Input: part model. Units: mm. Frame: model coordinates. A direction names the side the tool comes from. Coordinates: 2 decimals unless noted, no trailing zeros. Write each loop counter-clockwise with the first axis right and the second up, starting at its lowest first coordinate (ties: lowest second). Pieces come first, ordered by that corner, then holes. Notation, with made-up numbers: (76.25, -36) - (107.25, -36) arc R25 cw to (107.25, -12) - close; hole circle Ø9 at (58, -39). An arc over 180 degrees is marked (long way). Use a Markdown table: item, result. Add a question column.
Q1. Pin query (flat end, axial travel): P1, Ø1, axis at x = -8, y = 6, coming from the -Z side; P2, Ø8, axis at x = -5, z = -1, coming from the -Y side; P3, Ø1.5, axis at x = -14, z = -21, coming from the +Y side; P4, Ø0.9, axis at x = 3.5, y = 3.5, coming from the +Z side. Return the tip coordinate at first contact, or that it passes through.
Q2. Section query D-D (y = 5.5). Return the cut outline in (x, z), then the cut area to 3 significant figures.
Q3. Section query A-A (z = -25.5). Return the cut outline in (x, y), then the cut area to 3 significant figures.
Q4. Material intervals for probe 1 along X at (y, z) = (14.5, -9); probe 2 along X at (y, z) = (7, -21.5); probe 3 along Z at (x, y) = (-4.25, 9.5), sorted ascending. Write a range as from..to.
Q5. Mould query, pull axis X, two halves, no side actions, for faces 1 (the face through (-13, 8.85, -22)), 2 (the face through (5.347, 4, -22)), 3 (the face through (-5, 7, 0)). Classes: released by +X, released by -X, zero draft, split by the parting line, or undercut.
Q6. Set-up query: faces 4 (the face through (-5, 7, -12.127)), 5 (the face through (-14, 4, -14.627)), 6 (the face through (2.5, 7, -6)), 7 (the face through (-10.624, 4, -22)). Return all of +Z, -Z, +X, -X, +Y, -Y with unobstructed straight access to the full face (end or side cutting, diameter ignored); none if empty.
Q7. Section query B-B (y = 12.5). Return the cut outline in (x, z), then the cut area to 3 significant figures.
Q8. Section query C-C (x = -2.75). Return the cut outline in (y, z).
Autodesk Inventor part; units mm, degrees
ref_plane "YZ Plane" through (0, 0, 0) normal (1, 0, 0) x (0, 1, 0)
ref_plane "XZ Plane" through (0, 0, 0) normal (0, 1, 0) x (-1, 0, 0)
ref_plane "XY Plane" through (0, 0, 0) normal (0, 0, 1) x (1, 0, 0)
sketch "Sketch1" plane through (0, 0, 0) normal (0, 1, 0) x (-1, 0, 0)
  line L0 (0, 0) -> (10.127, 0)
  line L1 (10.127, 0) -> (10.127, -12.127)
  line L2 (10.127, -12.127) -> (0, -12.127)
  line L3 (0, -12.127) -> (0, 0)
  line L4 (-2.5, 2.5) -> (12.627, 2.5)
  line L5 (12.627, 2.5) -> (12.627, -14.627)
  line L6 (12.627, -14.627) -> (-2.5, -14.627)
  line L7 (-2.5, -14.627) -> (-2.5, 2.5)
  dimension "d5" = 10.127
  dimension "d6" = 12.127
  dimension "d7" = 2.5
  dimension "d8" = 2.5
  dimension "d9" = 2.5
  dimension "d10" = 2.5
extrude "Extrusion2" add sketch "Sketch1" along normal blind 15
sketch "Sketch3" plane through (2.5, 0, -14.627) normal (0, 0, -1) x (-1, 0, 0)
  line L0 (17.974, 0) -> (13.124, 0)
  line L1 (13.124, 0) -> (13.124, 8.85)
  line L2 (13.124, 8.85) -> (17.974, 8.85)
  line L3 (17.974, 8.85) -> (17.974, 0)
  line L4 (2.003, 0) -> (-2.847, 0)
  line L5 (-2.847, 0) -> (-2.847, 8.85)
  line L6 (-2.847, 8.85) -> (2.003, 8.85)
  line L7 (2.003, 8.85) -> (2.003, 0)
  line L8 (15.127, 0) -> (0, 0)
  line L9 (7.5635, 0) -> (7.5635, 15)
  line L10 (12.627, 15) -> (2.5, 15)
  dimension "d14" = 4.85
  dimension "d15" = 8.85
  dimension "d16" = 4.85
  dimension "d17" = 8.85
  dimension "d18" = 11.121
extrude "Extrusion3" add sketch "Sketch3" along normal blind 15
equation "\"d8\" = d7"
equation "\"d9\" = d7"
equation "\"d10\" = d7"
properties part number "motorMount"
Values follow:
| question | item | result |
|---|---|---|
| 1 | P1 | z = -14.63 |
| 1 | P2 | y = 0 |
| 1 | P3 | y = 8.85 |
| 1 | P4 | z = -14.63 |
| 2 | outline | (-15.47, -29.63) - (-10.62, -29.63) - (-10.62, -14.63) - (0.5, -14.63) - (0.5, -29.63) - (5.35, -29.63) - (5.35, -14.63) - (2.5, -14.63) - (2.5, 2.5) - (-12.63, 2.5) - (-12.63, -14.63) - (-15.47, -14.63) - close; hole (-10.13, -12.13) - (0, -12.13) - (0, 0) - (-10.13, 0) - close |
| 2 | area | 282 mm2 |
| 3 | outline | (-15.47, 0) - (-10.62, 0) - (-10.62, 8.85) - (-15.47, 8.85) - close; (0.5, 0) - (5.35, 0) - (5.35, 8.85) - (0.5, 8.85) - close |
| 3 | area | 85.8 mm2 |
| 4 | probe 1 | -12.63..-10.13, 0..2.5 |
| 4 | probe 2 | -15.47..-10.62, 0.5..5.35 |
| 4 | probe 3 | -14.63..-12.13, 0..2.5 |
| 5 | face 1 | zero draft |
| 5 | face 2 | released by +X |
| 5 | face 3 | undercut |
| 6 | face 4 | +Y, -Y |
| 6 | face 5 | +Z, -X, +Y, -Y |
| 6 | face 6 | +Z, +X, +Y, -Y |
| 6 | face 7 | -Z, +Y, -Y |
| 7 | outline | (-12.63, -14.63) - (2.5, -14.63) - (2.5, 2.5) - (-12.63, 2.5) - close; hole (-10.13, -12.13) - (0, -12.13) - (0, 0) - (-10.13, 0) - close |
| 7 | area | 136 mm2 |
| 8 | outline | (0, -14.63) - (15, -14.63) - (15, -12.13) - (0, -12.13) - close; (0, 0) - (15, 0) - (15, 2.5) - (0, 2.5) - close |
